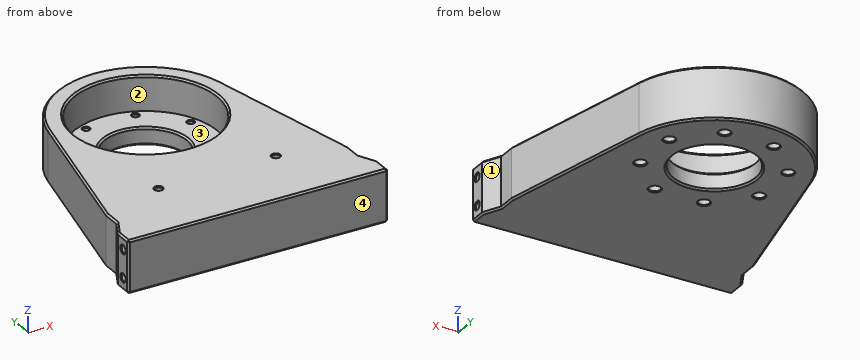
from build123d import *

# Parameters (mm, degrees)
SKETCH_1_W          = 149.5
SKETCH_1_H          = 165
EXTRUDE_1_DEPTH     = 30
CUT_EXTRUDE_1_DEPTH = 116.298796611
SKETCH_3_R          = 41
CUT_EXTRUDE_2_DEPTH = 20
SKETCH_4_R          = 23.75
CUT_EXTRUDE_3_DEPTH = 114.109736539
SKETCH_5_R          = 1.75
CUT_EXTRUDE_4_DEPTH = 116.298796611
SKETCH_6_R          = 3.1
CUT_EXTRUDE_5_DEPTH = 4
SKETCH_7_R          = 2.1
CUT_EXTRUDE_6_DEPTH = 8
CHAMFER_1_SIZE      = 0.5
CHAMFER_2_SIZE      = 1
CHAMFER_3_SIZE      = 0.5
CUT_EXTRUDE_7_DEPTH = 116.298796611
CHAMFER_4_SIZE      = 1
SKETCH_9_R          = 2.1
CUT_EXTRUDE_8_DEPTH = 8
CHAMFER_5_SIZE      = 0.5


with BuildPart() as part:
    # 草图1 → 凸台-拉伸1 (new body)
    with BuildSketch(Plane.XY):
        Rectangle(SKETCH_1_W, SKETCH_1_H)
    extrude(amount=EXTRUDE_1_DEPTH)

    # 草图2 → 切除-拉伸1 (cut, through all)
    with BuildSketch(Plane.XY.offset(30)):
        Polygon((-74.75, 82.5), (-74.75, -72.5), (-69.75, -62.5), (-69.75, 82.5), align=None)
        Polygon((69.75, 82.5), (74.75, 82.5), (74.75, -72.5), (69.75, -62.5), align=None)
    extrude(amount=-CUT_EXTRUDE_1_DEPTH, mode=Mode.SUBTRACT)

    # 草图3 → 切除-拉伸2 (cut)
    with BuildSketch(Plane.XY.offset(30)):
        with Locations((0, 27.5)):
            Circle(SKETCH_3_R)
    extrude(amount=-CUT_EXTRUDE_2_DEPTH, mode=Mode.SUBTRACT)

    # 草图4 → 切除-拉伸3 (cut, through all)
    with BuildSketch(Plane.XY.offset(10)):
        with Locations((0, 27.5)):
            Circle(SKETCH_4_R)
    extrude(amount=-CUT_EXTRUDE_3_DEPTH, mode=Mode.SUBTRACT)

    # 草图5 → 切除-拉伸4 (cut, through all)
    with BuildSketch(Plane(origin=(0, 0, 0), x_dir=(-1, 0, 0), z_dir=(0, 0, -1))):
        with Locations((14.159286998, 61.683542703)):
            Circle(SKETCH_5_R)
        with Locations((34.183542703, 41.659286998)):
            Circle(SKETCH_5_R)
        with Locations((34.183542703, 13.340713002)):
            Circle(SKETCH_5_R)
        with Locations((14.159286998, -6.683542703)):
            Circle(SKETCH_5_R)
        with Locations((-14.159286998, -6.683542703)):
            Circle(SKETCH_5_R)
        with Locations((-34.183542703, 13.340713002)):
            Circle(SKETCH_5_R)
        with Locations((-34.183542703, 41.659286998)):
            Circle(SKETCH_5_R)
        with Locations((-14.159286998, 61.683542703)):
            Circle(SKETCH_5_R)
    extrude(amount=-CUT_EXTRUDE_4_DEPTH, mode=Mode.SUBTRACT)

    # 草图6 → 切除-拉伸5 (cut)
    with BuildSketch(Plane(origin=(0, 0, 0), x_dir=(-1, 0, 0), z_dir=(0, 0, -1))):
        with Locations((14.159286998, 61.683542703)):
            Circle(SKETCH_6_R)
        with Locations((34.183542703, 41.659286998)):
            Circle(SKETCH_6_R)
        with Locations((34.183542703, 13.340713002)):
            Circle(SKETCH_6_R)
        with Locations((14.159286998, -6.683542703)):
            Circle(SKETCH_6_R)
        with Locations((-14.159286998, -6.683542703)):
            Circle(SKETCH_6_R)
        with Locations((-34.183542703, 13.340713002)):
            Circle(SKETCH_6_R)
        with Locations((-34.183542703, 41.659286998)):
            Circle(SKETCH_6_R)
        with Locations((-14.159286998, 61.683542703)):
            Circle(SKETCH_6_R)
    extrude(amount=-CUT_EXTRUDE_5_DEPTH, mode=Mode.SUBTRACT)

    # 草图7 → 切除-拉伸6 (cut)
    with BuildSketch(Plane(origin=(74.75, 0, 0), x_dir=(0, 0, -1), z_dir=(1, 0, 0))):
        with Locations(Location((-23, -77.5, 0), (0, 0, 90))):
            Circle(SKETCH_7_R)
        with Locations(Location((-7, -77.5, 0), (0, 0, 270))):
            Circle(SKETCH_7_R)
    cut_extrude_6 = extrude(amount=-CUT_EXTRUDE_6_DEPTH, mode=Mode.SUBTRACT)

    # 镜向1: 切除-拉伸6 across plane
    add(cut_extrude_6.mirror(Plane(origin=(0, 0, 0), x_dir=(0, 0, 1), z_dir=(1, 0, 0))), mode=Mode.SUBTRACT)

    # 倒角1
    chamfer_1_edges = [part.edges().sort_by_distance(p)[0] for p in [
        (74.75, -79.6, 23),
        (74.75, -75.4, 7),
        (-74.75, -79.6, 23),
        (-74.75, -75.4, 7),
    ]]
    chamfer(chamfer_1_edges, length=CHAMFER_1_SIZE)

    # 倒角2
    chamfer_2_edges = [part.edges().sort_by_distance(p)[0] for p in [
        (-41, 27.5, 30),
        (-23.75, 27.5, 0),
        (-23.75, 27.5, 10),
    ]]
    chamfer(chamfer_2_edges, length=CHAMFER_2_SIZE)

    # 倒角3
    chamfer_3_edges = [part.edges().sort_by_distance(p)[0] for p in [
        (-32.433542703, 41.659286998, 4),
        (-31.083542703, 41.659286998, 0),
        (-32.433542703, 13.340713002, 4),
        (-31.083542703, 13.340713002, 0),
        (-12.409286998, -6.683542703, 4),
        (-11.059286998, -6.683542703, 0),
        (15.909286998, -6.683542703, 4),
        (17.259286998, -6.683542703, 0),
        (35.933542703, 13.340713002, 4),
        (37.283542703, 13.340713002, 0),
        (35.933542703, 41.659286998, 4),
        (37.283542703, 41.659286998, 0),
        (15.909286998, 61.683542703, 4),
        (17.259286998, 61.683542703, 0),
        (-12.409286998, 61.683542703, 4),
        (-11.059286998, 61.683542703, 0),
        (-32.433542703, 41.659286998, 10),
        (-32.433542703, 13.340713002, 10),
        (-12.409286998, -6.683542703, 10),
        (15.909286998, -6.683542703, 10),
        (35.933542703, 13.340713002, 10),
        (35.933542703, 41.659286998, 10),
        (15.909286998, 61.683542703, 10),
        (-12.409286998, 61.683542703, 10),
    ]]
    chamfer(chamfer_3_edges, length=CHAMFER_3_SIZE)

    # 草图8 → 切除-拉伸7 (cut, through all)
    with BuildSketch(Plane.XY.offset(30)):
        with BuildLine():
            Line((-69.75, -52.5), (-49.816857163, 38.421572339))
            ThreePointArc((-49.816857163, 38.421572339), (0, 78.5), (49.816857163, 38.421572339))
            Line((49.816857163, 38.421572339), (69.75, -52.5))
            Line((69.75, -52.5), (69.75, 82.5))
            Line((69.75, 82.5), (-69.75, 82.5))
            Line((-69.75, 82.5), (-69.75, -52.5))
        make_face()
    extrude(amount=-CUT_EXTRUDE_7_DEPTH, mode=Mode.SUBTRACT)

    # 倒角4
    chamfer_4_edges = [part.edges().sort_by_distance(p)[0] for p in [
        (-74.75, -77.5, 0),
        (0, -82.5, 30),
        (-74.75, -77.5, 30),
        (-69.75, -57.5, 0),
        (-72.25, -67.5, 0),
        (-72.25, -67.5, 30),
        (-69.75, -57.5, 30),
        (69.75, -57.5, 30),
        (69.75, -57.5, 0),
        (59.783428582, -7.03921383, 0),
        (0, 78.5, 0),
        (-59.783428582, -7.03921383, 0),
        (-59.783428582, -7.03921383, 30),
        (0, 78.5, 30),
        (59.783428582, -7.03921383, 30),
        (72.25, -67.5, 0),
        (72.25, -67.5, 30),
        (74.75, -77.5, 30),
        (0, -82.5, 0),
        (74.75, -77.5, 0),
        (74.75, -82.5, 15),
        (-74.75, -82.5, 15),
    ]]
    chamfer(chamfer_4_edges, length=CHAMFER_4_SIZE)

    # 草图9 → 切除-拉伸8 (cut)
    with BuildSketch(Plane(origin=(0, 0, 30), x_dir=(-1, 0, 0), z_dir=(0, 0, -1))):
        with Locations((-33.75, -42.5)):
            Circle(SKETCH_9_R)
        with Locations((33.75, -42.5)):
            Circle(SKETCH_9_R)
    extrude(amount=CUT_EXTRUDE_8_DEPTH, mode=Mode.SUBTRACT)

    # 倒角5
    chamfer_5_edges = [part.edges().sort_by_distance(p)[0] for p in [
        (35.85, -42.5, 30),
        (-31.65, -42.5, 30),
    ]]
    chamfer(chamfer_5_edges, length=CHAMFER_5_SIZE)


solid = part.part
Check sheet for the modelled part. Datum: model origin and axes. Units: mm. Face numbers are marked on the shaded views. Coordinates: 2 decimals unless noted, no trailing zeros. Loops run counter-clockwise (first coordinate to the right, second up) from the corner with the lowest first, then second, coordinate; pieces in that order, holes last. Notation, with made-up numbers: (12.5, 72.25) -> (71.5, 72.25) arc R23 ccw to (71.5, 92.25) -> close; hole circle Ø3 at (-9.5, -11). An arc over 180 degrees is marked (long way). Write item = value, one per line. Start each with the question number.
1. Draft check along Y on the marked faces 1, 2, 3 and 4. Enter one of: released by +Y, released by -Y, zero draft, split by the parting line, or undercut.
2. Section check A-A on z = 15. Record the cut outline in (x, y), then the cut area to 3 significant figures.
3. Section check B-B on y = -42.5. Record the cut outline in (x, z), then the cut area to 3 significant figures.
4. Depth check by flat-ended pin: P1, Ø6, axis at y = 43, z = 4.5, coming from the +X side; P2, Ø3, axis at y = 23, z = 24.5, coming from the +X side; P3, Ø6.5, axis at y = -77.5, z = 23, coming from the +X side; P4, Ø6, axis at x = -10, z = 20, coming from the +Y side. Enter the tip coordinate at first touch or a pass-through.
5. Material ranges on line 1 (Z direction, x = -70, y = -77.5); line 2 (X direction, y = 44, z = 3.5); line 3 (Y direction, x = -1.5, z = 19), recorded low to high.
Responses:
q1.face_1 = released by +Y
q1.face_2 = undercut
q1.face_3 = undercut
q1.face_4 = released by -Y
q2.outline = (-74.75, -81.5) -> (-73.75, -82.5) -> (73.75, -82.5) -> (74.75, -81.5) -> (74.75, -72.5) -> (69.75, -62.5) -> (69.75, -52.5) -> (49.82, 38.42) arc R51 ccw to (-49.82, 38.42) -> (-69.75, -52.5) -> (-69.75, -62.5) -> (-74.75, -72.5) -> close; hole circle Ø82 at (0, 27.5)
q2.area = 12,900 mm2
q3.outline = (-67.56, 1) -> (-66.53, 0) -> (66.53, 0) -> (67.56, 1) -> (67.56, 29) -> (66.53, 30) -> (36.35, 30) -> (35.85, 29.5) -> (35.85, 22) -> (31.65, 22) -> (31.65, 29.5) -> (31.15, 30) -> (-31.15, 30) -> (-31.65, 29.5) -> (-31.65, 22) -> (-35.85, 22) -> (-35.85, 29.5) -> (-36.35, 30) -> (-66.53, 30) -> (-67.56, 29) -> close
q3.area = 3,980 mm2
q4.P1 = 49.44
q4.P2 = 53.53
q4.P3 = 74.75
q4.P4 = 78.02
q5.line_1 = 0 to 4.9, 9.1 to 20.9, 25.1 to 30
q5.line_2 = -48.26 to -36.22, -32.15 to -17.08, 17.08 to 32.15, 36.22 to 48.26
q5.line_3 = -82.5 to -13.47, 68.47 to 78.48
